Input: part model. Units: mm. Frame: model coordinates. Coordinates: 2 decimals unless noted, no trailing zeros. Order: outer loops, then holes, each group sorted by start corner. A loop starts at its lowest first (then second) coordinate and runs counter-clockwise, first axis right, second up. Notation, with made-up numbers: M 63,6 L 96,6 A21 cw 96,24 Z; hole C 30.25,79.25 d9. An arc over 180 degrees is marked long. Answer in a Markdown table with one row per item.
from build123d import *

# Parameters (mm, degrees)
F0_W     = 25.35
F0_H     = 25.35
F1_DEPTH = 5.5


with BuildPart() as f1:
    # F0 (on Top) → F1 (new body)
    with BuildSketch(Plane.XY):
        Polygon((47.5, 27.675), (-47.5, 27.675), (-92.037046, 1.961524), (-62.037046, -50), (62.037046, -50), (92.037046, 1.961524), (74.716538, 11.961524), align=None)
        Rectangle(F0_W, F0_H, mode=Mode.SUBTRACT)
    extrude(amount=F1_DEPTH)


solid = f1.part
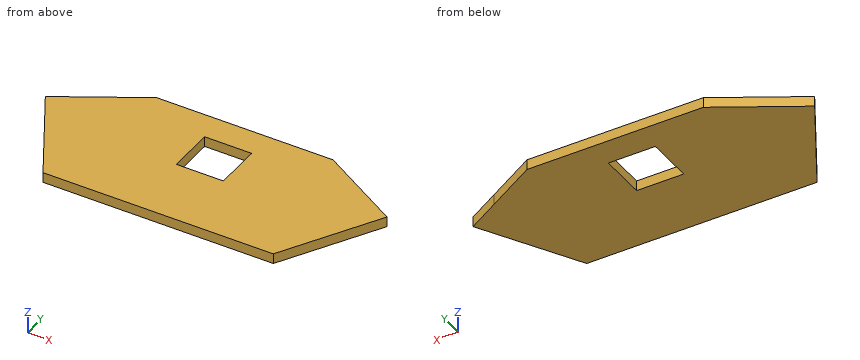
1) Material intervals for probe 1 along Y at (x, z) = (-4.5, 2.1) (3 decimals); probe 2 along X at (y, z) = (0, 3.7) (3 decimals); probe 3 along X at (y, z) = (-4, 0.7) (3 decimals), sorted ascending.
Resolved:
| item | result |
|---|---|
| probe 1 | y = -50 to -12.675, 12.675 to 27.675 |
| probe 2 | x = -90.905 to -12.675, 12.675 to 90.905 |
| probe 3 | x = -88.595 to -12.675, 12.675 to 88.595 |
2) Cut plane C-C, the plane y = 22.5. Output: boundary loops of the cut face in (x, z).
Resolved:
| item | result |
|---|---|
| outline | M -56.46,0 L 56.46,0 L 56.46,5.5 L -56.46,5.5 Z |
3) Cut plane B-B, the plane z = 3.9. Output: boundary loops of the cut face in (x, y) (3 decimals), and give its area (3 significant figures).
Resolved:
| item | result |
|---|---|
| outline | M -92.037,1.962 L -62.037,-50 L 62.037,-50 L 92.037,1.962 L 47.5,27.675 L -47.5,27.675 Z; hole M -12.675,-12.675 L 12.675,-12.675 L 12.675,12.675 L -12.675,12.675 Z |
| area | 11,000 mm2 |
4) Cut plane A-A, the plane x = -4. Output: boundary loops of the cut face in (y, z) (3 decimals), and give its area (3 significant figures).
Resolved:
| item | result |
|---|---|
| outline | M -50,0 L -12.675,0 L -12.675,5.5 L -50,5.5 Z; M 12.675,0 L 27.675,0 L 27.675,5.5 L 12.675,5.5 Z |
| area | 288 mm2 |
5) Cut plane D-D, the plane x = 71.5. Output: boundary loops of the cut face in (y, z), and give its area (3 significant figures).
Resolved:
| item | result |
|---|---|
| outline | M -33.61,0 L 13.82,0 L 13.82,5.5 L -33.61,5.5 Z |
| area | 261 mm2 |
6) Contact query for flat-ended pins moving along their axis: pin 1 (8 mm diameter, centred on x = -65, y = -8.5, fed in from -Z); pin 2 (3 mm diameter, centred on y = 5, z = 1.5, fed in from -X). Output: stop coordinate, or through.
Resolved:
| item | result |
|---|---|
| pin 1 | stops at z = 0 |
| pin 2 | stops at x = -89.37 |
